```python
from build123d import *

# Parameters (mm, degrees)
SKETCH1_R           = 3
BOSS_EXTRUDE1_DEPTH = 20
SKETCH2_R           = 1
BOSS_EXTRUDE2_DEPTH = 20


with BuildPart() as part:
    # Sketch1 → Boss-Extrude1 (new body)
    with BuildSketch(Plane.XY):
        Circle(SKETCH1_R)
    extrude(amount=BOSS_EXTRUDE1_DEPTH)

    # Sketch2 → Boss-Extrude2 (add)
    with BuildSketch(Plane.XY.offset(20)):
        with Locations((-2, 0)):
            Circle(SKETCH2_R)
        with Locations((2, 0)):
            Circle(SKETCH2_R)
    extrude(amount=BOSS_EXTRUDE2_DEPTH)


solid = part.part
```
Source: CAD feature listing. Evaluate the final solid. Frame: model axes, mm. A direction names the side the tool comes from. Round coordinates to 2 decimals unless told otherwise and drop trailing zeros. Order: outer loops, then holes, each group sorted by start corner. A loop starts at its lowest first (then second) coordinate and runs counter-clockwise, first axis right, second up. Notation, with made-up numbers: (84, -2) -> (136, -2) arc R29 ccw to (136, 28) -> close; hole circle Ø7 at (-29.5, -25.5). An arc over 180 degrees is marked (long way). Use CSV: the item, a comma, the result in double quotes.
(1) Section C-C on y = -0.65. Return the cut outline in (x, z), and give its area (3 significant figures).
Report:
outline,"(-2.93, 0) -> (2.93, 0) -> (2.93, 20) -> (2.76, 20) -> (2.76, 40) -> (1.24, 40) -> (1.24, 20) -> (-1.24, 20) -> (-1.24, 40) -> (-2.76, 40) -> (-2.76, 20) -> (-2.93, 20) -> close"
area,"178 mm^2"
(2) Section D-D on z = 11. Return the cut outline in (x, y), and give its area (3 significant figures).
Report:
outline,"circle Ø6 at (0, 0)"
area,"28.3 mm^2"
(3) Access query for faces 4 (the face through (-2.8, -0.6, 29.9)), 5 (the face through (-2, 0, 40)). Directions: +Z, -Z, +X, -X, +Y, -Y. A direction counts if a zero-diameter tool reaches every point of the face in a straight line with its end or side. Return the directions, or none.
Report:
face 4,"+Z"
face 5,"+Z, +X, -X, +Y, -Y"
(4) Section A-A on z = 25. Return the cut outline in (x, y), and give its area (3 significant figures).
Report:
outline,"circle Ø2 at (-2, 0); circle Ø2 at (2, 0)"
area,"6.28 mm^2"
(5) Pull-direction query (X, two-part tool) for faces 1 (the face through (0, 0, 20)), 2 (the face through (2, 0, 40)), 3 (the face through (-3, 0, 10)); classes: +X half, -X half, draft (parallel to the pull), parting line (faces both ways), or undercut.
Report:
face 1,"undercut"
face 2,"draft"
face 3,"parting line"
(6) Ray query, L1, parallel to X at y = -0.1, z = 22; L2, parallel to Z at x = -0.2, y = -0.5; L3, parallel to X at y = 0.6, z = 28. Return the intervals inside material, ascending.
Report:
L1,"-2.99 to -1.01, 1.01 to 2.99"
L2,"0 to 20"
L3,"-2.8 to -1.2, 1.2 to 2.8"
(7) Section B-B on x = 0. Return the cut outline in (y, z).
Report:
outline,"(-3, 0) -> (3, 0) -> (3, 20) -> (-3, 20) -> close"
